Geometry check sheet. Reference: the model listing, model coordinates, mm. Face numbers are marked on the shaded views. A direction names the side the tool comes from. Give positions to 0.01 mm unless a question says otherwise; leave off trailing zeros. Loops run counter-clockwise (first coordinate to the right, second up) from the corner with the lowest first, then second, coordinate; pieces in that order, holes last. Notation, with made-up numbers: (-21, 39.25) -> (-7, 39.25) arc R36 ccw to (-7, 78.25) -> close; hole circle Ø3 at (-28, 88.5). An arc over 180 degrees is marked (long way). Write each question's results on one line, items separated by ' | '. Start each with the question number.
1) Sectioned sample at A-A on z = 6. Record the cut outline in (x, y).
2) Depth check by flat-ended pin: pin 1 (3 mm diameter, centred on x = 12, y = 10.5, fed in from +Z). Enter the tip coordinate at first touch or a pass-through.
3) Set-up check for the marked faces 3 and 4: record each of +Z, -Z, +X, -X, +Y, -Y from which the full face is reachable in a straight line by a thin tool's end or side.
4) Sectioned sample at B-B on x = -20. Record the cut outline in (y, z), then the cut area to 3 significant figures.
5) Scan lines: line 1 (X direction, y = -11.5, z = 5.5); line 2 (Y direction, x = -76.5, z = 14.25); line 3 (Z direction, x = -77, y = 23.5). Record each from-to range of solid material in increasing order. Write a range as from..to.
6) Draft check along Y on the marked faces 1 and 2. Enter one of: pulls with the +Y half, pulls with the -Y half, needs draft (parallel to the pull), parting line crosses it, or undercut.
7) Sectioned sample at C-C on y = -35. Record the cut outline in (x, z), then the cut area to 3 significant figures.
```python
from build123d import *

# Parameters (mm, degrees)
F0_W     = 198
F0_H     = 82
F1_DEPTH = 15
F2_T     = -2.5
F3_SIZE  = 0.2


with BuildPart() as f1:
    # F0 (on Top) → F1 (new body)
    with BuildSketch(Plane.XY):
        Rectangle(F0_W, F0_H)
    extrude(amount=F1_DEPTH)

    # F2
    f2_openings = [f1.faces().sort_by_distance(p)[0] for p in [
        (0, 0, 15),
    ]]
    offset(amount=F2_T, openings=f2_openings)

    # F3
    f3_edges = [f1.edges().sort_by_distance(p)[0] for p in [
        (99, 41, 7.5),
        (99, -41, 7.5),
        (-99, -41, 7.5),
        (0, -41, 0),
        (0, -41, 15),
        (0, 41, 15),
        (-99, 0, 15),
        (99, 0, 0),
        (99, 0, 15),
        (-96.5, 38.5, 8.75),
        (0, -38.5, 15),
        (0, 38.5, 2.5),
        (0, 38.5, 15),
        (-96.5, 0, 2.5),
        (-96.5, 0, 15),
        (96.5, 0, 15),
        (-99, 41, 7.5),
        (0, 41, 0),
        (-99, 0, 0),
        (-96.5, -38.5, 8.75),
        (96.5, -38.5, 8.75),
        (96.5, 38.5, 8.75),
        (0, -38.5, 2.5),
        (96.5, 0, 2.5),
    ]]
    chamfer(f3_edges, length=F3_SIZE)


solid = f1.part
```
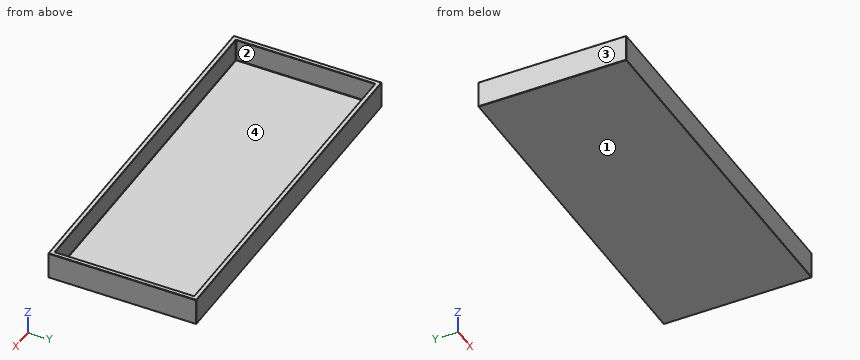
Result:
1) outline: (-99, -40.8) -> (-98.8, -41) -> (98.8, -41) -> (99, -40.8) -> (99, 40.8) -> (98.8, 41) -> (-98.8, 41) -> (-99, 40.8) -> close; hole (-96.5, -38.3) -> (-96.3, -38.5) -> (96.3, -38.5) -> (96.5, -38.3) -> (96.5, 38.3) -> (96.3, 38.5) -> (-96.3, 38.5) -> (-96.5, 38.3) -> close
2) pin 1: z = 2.5
3) face 3: +Z, -Z, -X, +Y, -Y | face 4: +Z
4) outline: (-41, 0.2) -> (-40.8, 0) -> (40.8, 0) -> (41, 0.2) -> (41, 14.8) -> (40.8, 15) -> (38.7, 15) -> (38.5, 14.8) -> (38.5, 2.7) -> (38.3, 2.5) -> (-38.3, 2.5) -> (-38.5, 2.7) -> (-38.5, 14.8) -> (-38.7, 15) -> (-40.8, 15) -> (-41, 14.8) -> close | area: 267 mm^2
5) line 1: -99..-96.5, 96.5..99 | line 2: -41..-38.5, 38.5..41 | line 3: 0..2.5
6) face 1: needs draft | face 2: undercut
7) outline: (-99, 0.2) -> (-98.8, 0) -> (98.8, 0) -> (99, 0.2) -> (99, 14.8) -> (98.8, 15) -> (96.7, 15) -> (96.5, 14.8) -> (96.5, 2.7) -> (96.3, 2.5) -> (-96.3, 2.5) -> (-96.5, 2.7) -> (-96.5, 14.8) -> (-96.7, 15) -> (-98.8, 15) -> (-99, 14.8) -> close | area: 557 mm^2
